```python
from build123d import *

# Parameters (mm, degrees)
F0_R     = 12.254349
F1_DEPTH = 50.8
F2_R     = 8.291725
F2_R_2   = 8.507614
F3_DEPTH = 10.16
F5_DEPTH = 6.35


with BuildPart() as f1:
    # F0 (on Front) → F1 (new body)
    with BuildSketch(Plane.XZ):
        with BuildLine():
            Line((76.394036, 56.497514), (27.739568, 56.497514))
            ThreePointArc((27.739568, 56.497514), (-0.754078, 84.226831), (-27.69857, 54.989916))
            Line((-27.69857, 54.989916), (-74.78258, 54.989916))
            Line((-74.78258, 54.989916), (-74.78258, 17.613143))
            Line((-74.78258, 17.613143), (-27.358174, 17.613143))
            Line((-27.358174, 17.613143), (-27.358174, 0))
            Line((-27.358174, 0), (0, 0))
            Line((0, 0), (31.513482, 0))
            Line((31.513482, 0), (31.513482, 19.248471))
            Line((31.513482, 19.248471), (76.394036, 19.248471))
            Line((76.394036, 19.248471), (76.394036, 56.497514))
        make_face()
        with Locations((0, 56.497514)):
            Circle(F0_R, mode=Mode.SUBTRACT)
    extrude(amount=F1_DEPTH)

    # F2 (on Front) → F3 (join)
    with BuildSketch(Plane.XZ):
        with BuildLine():
            Line((-74.914232, -26.959702), (-15.175805, -89.64081))
            ThreePointArc((-15.175805, -89.64081), (-0.268287, -96.139845), (14.800677, -90.024463))
            Line((14.800677, -90.024463), (76.250419, -28.766453))
            Line((76.250419, -28.766453), (76.250419, 21.220267))
            Line((76.250419, 21.220267), (-74.914232, 21.220267))
            Line((-74.914232, 21.220267), (-74.914232, -26.959702))
        make_face()
        with Locations((-44.199497, -24.952203)):
            Circle(F2_R, mode=Mode.SUBTRACT)
        with Locations((38.710192, -23.948461)):
            Circle(F2_R_2, mode=Mode.SUBTRACT)
    extrude(amount=F3_DEPTH)

    # F4 (on Right) → F5 (join, symmetric)
    with BuildSketch(Plane.YZ):
        Polygon((-10.954797, 0), (-50.737962, 0), (-10.954797, -72.062641), align=None)
    extrude(amount=F5_DEPTH, both=True)


solid = f1.part
```
Can you work these out from the model? Positions are in its coordinate system, mm. A direction names the side the tool comes from. Coordinates: 2 decimals unless noted, no trailing zeros. Loops run counter-clockwise (first coordinate to the right, second up) from the corner with the lowest first, then second, coordinate; pieces in that order, holes last. Notation, with made-up numbers: (75, -7) - (98, -7) arc R13 cw to (98, 18) - close; hole circle Ø4 at (-29.75, 26). An arc over 180 degrees is marked (long way). Use a Markdown table: item, result.
Item 1: I want a section at B-B on z = -49.5. Please give me the cut outline in (x, y), and give its area (3 significant figures).
Numbers:
| item | result |
|---|---|
| outline | (-53.43, -10.16) - (55.45, -10.16) - (55.45, 0) - (-53.43, 0) - close; (-6.35, -23.41) - (6.35, -23.41) - (6.35, -10.95) - (-6.35, -10.95) - close |
| area | 1,260 mm2 |
Item 2: We'd pull the mould along Y, two halves only. Please class faces 4 (the face through (-36.54, -5.01, -28.13)), 5 (the face through (0, -10.955, -37)), 6 (the face through (0, 0, -5)): released by +Y, released by -Y, zero draft, split by the parting line, or undercut.
Numbers:
| item | result |
|---|---|
| face 4 | zero draft |
| face 5 | undercut |
| face 6 | released by +Y |
Item 3: I want a section at D-D on z = -5. Please give me the cut outline in (x, y).
Numbers:
| item | result |
|---|---|
| outline | (-74.91, -10.16) - (76.25, -10.16) - (76.25, 0) - (-74.91, 0) - close; (-6.35, -47.98) - (6.35, -47.98) - (6.35, -10.95) - (-6.35, -10.95) - close |
Item 4: If I drill on probe 1 along X at (y, z) = (-9, -18.5); probe 2 along Z at (x, y) = (4.5, -39); probe 3 along Z at (x, y) = (63.5, -20), over which ranges is the centre line in solid material (lowest first)? Write a range as from..to.
Numbers:
| item | result |
|---|---|
| probe 1 | x = -74.91..-49.41, -38.99..32.18, 45.24..76.25 |
| probe 2 | z = -21.26..45.1, 67.9..83.87 |
| probe 3 | z = 19.25..56.5 |
Item 5: For faces 1 (the face through (6.35, -22, -20)), 2 (the face through (-6.35, -22, -20)), 3 (the face through (-0.502, -5.009, -96.136)), which set-ups out of +Z, -Z, +X, -X, +Y, -Y let a thin tool reach every point of the face, with its end or its side?
Numbers:
| item | result |
|---|---|
| face 1 | -Z, +X, -Y |
| face 2 | -Z, -X, -Y |
| face 3 | -Z, +Y, -Y |
Item 6: I want a section at A-A on x = 0. Please give me the cut outline in (y, z).
Numbers:
| item | result |
|---|---|
| outline | (-50.8, 0) - (-50.74, 0) - (-10.95, -72.06) - (-10.95, 0) - (-10.16, 0) - (-10.16, -96.14) - (0, -96.14) - (0, 44.24) - (-50.8, 44.24) - close; (-50.8, 68.75) - (0, 68.75) - (0, 84.24) - (-50.8, 84.24) - close |
Item 7: Will these pins go through, and if not, where does the flat tip stop? pin 1 (23.5 mm diameter, centred on x = -47, y = -14, fed in from +Z); pin 2 (1 mm diameter, centred on x = -21, y = -36, fed in from -Z); pin 3 (20.5 mm diameter, centred on x = -42, y = -25.5, fed in from -Z); pin 4 (3 mm diameter, centred on y = -42.5, z = -21.5, fed in from +X).
Numbers:
| item | result |
|---|---|
| pin 1 | stops at z = 54.99 |
| pin 2 | stops at z = 0 |
| pin 3 | stops at z = 17.61 |
| pin 4 | passes through |
Item 8: I want a section at C-C on y = -39.5. Please give me the cut outline in (x, z).
Numbers:
| item | result |
|---|---|
| outline | (-74.78, 17.61) - (-27.36, 17.61) - (-27.36, 0) - (-6.35, 0) - (-6.35, -20.36) - (6.35, -20.36) - (6.35, 0) - (31.51, 0) - (31.51, 19.25) - (76.39, 19.25) - (76.39, 56.5) - (27.74, 56.5) arc R27.74 ccw (long way) to (-27.7, 54.99) - (-74.78, 54.99) - close; hole circle Ø24.51 at (0, 56.5) |
